from build123d import *

# Parameters (mm, degrees)
BOSS_EXTRUDE1_DEPTH = 3.175
BOSS_EXTRUDE2_DEPTH = 3.175
CUT_EXTRUDE2_DEPTH  = 159.172640977
CIRPATTERN1_COUNT   = 6
SKETCH4_R           = 8.001
CUT_EXTRUDE3_DEPTH  = 3.175
BOSS_EXTRUDE3_DEPTH = 2.54
CIRPATTERN2_COUNT   = 6


with BuildPart() as part:
    # Sketch1 → Boss-Extrude1 (new body)
    with BuildSketch(Plane(origin=(0, 0, 0), x_dir=(1, 0, 0), z_dir=(0, 1, 0))):
        Polygon((55.499999998, -96.128819817), (110.999999996, 0), (55.499999998, 96.128819817), (-55.499999998, 96.128819817), (-110.999999996, 0), (-55.499999998, -96.128819817), align=None)
    extrude(amount=BOSS_EXTRUDE1_DEPTH)

    # Sketch2 → Boss-Extrude2 (add)
    with BuildSketch(Plane(origin=(0, 0, 0), x_dir=(1, 0, 0), z_dir=(0, 1, 0))):
        with BuildLine():
            ThreePointArc((23.622499999, 104.383819817), (24.109685288, 98.980852172), (19.494999999, 96.128819817))
            Line((19.494999999, 96.128819817), (36.004999999, 96.128819817))
            ThreePointArc((36.004999999, 96.128819817), (31.39031471, 98.980852172), (31.877499999, 104.383819817))
            ThreePointArc((31.877499999, 104.383819817), (32.364685288, 109.786787461), (27.749999999, 112.638819817))
            ThreePointArc((27.749999999, 112.638819817), (23.13531471, 109.786787461), (23.622499999, 104.383819817))
        make_face()
    boss_extrude2 = extrude(amount=BOSS_EXTRUDE2_DEPTH)

    # Sketch2<3> → Cut-Extrude2 (cut, through all)
    with BuildSketch(Plane(origin=(0, 0, 0), x_dir=(1, 0, 0), z_dir=(0, 1, 0))):
        with BuildLine():
            Line((-19.494999999, 96.128819817), (-36.004999999, 96.128819817))
            ThreePointArc((-36.004999999, 96.128819817), (-31.39031471, 93.276787461), (-31.877499999, 87.873819817))
            ThreePointArc((-31.877499999, 87.873819817), (-32.364685288, 82.470852172), (-27.749999999, 79.618819817))
            ThreePointArc((-27.749999999, 79.618819817), (-23.13531471, 82.470852172), (-23.622499999, 87.873819817))
            ThreePointArc((-23.622499999, 87.873819817), (-24.109685288, 93.276787461), (-19.494999999, 96.128819817))
        make_face()
    cut_extrude2 = extrude(amount=CUT_EXTRUDE2_DEPTH, mode=Mode.SUBTRACT)

    # CirPattern1: Boss-Extrude2, Cut-Extrude2 ×6 about axis
    cirpattern1_axis = Axis((0, 0, 0), (0, 1, 0))
    add([boss_extrude2.rotate(cirpattern1_axis, i * 360 / CIRPATTERN1_COUNT) for i in range(1, CIRPATTERN1_COUNT)])
    add([cut_extrude2.rotate(cirpattern1_axis, i * 360 / CIRPATTERN1_COUNT) for i in range(1, CIRPATTERN1_COUNT)], mode=Mode.SUBTRACT)

    # Sketch4 → Cut-Extrude3 (cut)
    with BuildSketch(Plane(origin=(0, 3.175, 0), x_dir=(1, 0, 0), z_dir=(0, 1, 0))):
        with Locations(Location((0, 0, 0), (0, 0, 270))):
            Circle(SKETCH4_R)
    extrude(amount=-CUT_EXTRUDE3_DEPTH, mode=Mode.SUBTRACT)

    # Sketch5 → Boss-Extrude3 (add)
    with BuildSketch(Plane(origin=(0, 3.175, 0), x_dir=(1, 0, 0), z_dir=(0, 1, 0))):
        Polygon((-8.429069256, -1.402423789), (-84.749999997, -45.466333697), (-83.249999997, -48.064409908), (-6.929069256, -4.0005), align=None)
        Polygon((-6.929069256, -4.0005), (-83.249999997, -48.064409908), (-81.749999997, -50.66248612), (-5.429069256, -6.598576211), align=None)
    boss_extrude3 = extrude(amount=BOSS_EXTRUDE3_DEPTH)

    # CirPattern2: Boss-Extrude3 ×6 about axis
    cirpattern2_axis = Axis((0, 0, 0), (0, 1, 0))
    for i in range(1, CIRPATTERN2_COUNT):
        add(boss_extrude3.rotate(cirpattern2_axis, i * 360 / CIRPATTERN2_COUNT))


solid = part.part
Verification items for the finished model (mm, model axes). A direction names the side the tool comes from. Coordinates: 2 decimals unless noted, no trailing zeros. Write each loop counter-clockwise with the first axis right and the second up, starting at its lowest first coordinate (ties: lowest second). Pieces come first, ordered by that corner, then holes. Notation, with made-up numbers: (65.5, 21.5) -> (121.5, 21.5) arc R23 cw to (121.5, 30.5) -> close; hole circle Ø4 at (50, 22.25). An arc over 180 degrees is marked (long way). One line per item, written item: value. Start each with the question number.
Q1. Cross-section at A-A on x = 43.5. Enter the section's corners in (y, z) (3 decimals), and give its area (3 significant figures).
Q2. Access from +Z, -Z, +X, -X, +Y, -Y to the whole of each face (thin tool, end or side, straight path). Record for faces 1 (the flat face through (-32, 3.175, 58)), 2 (the flat face through (60.306, 1.565, 87.805)), 3 (the flat face through (-43.055, 4.427, -28.322)).
Q3. Thickness scan on L1, parallel to X at y = 1.7, z = 0; L2, parallel to Z at x = 0, y = 0.7; L3, parallel to Y at x = 90.5, z = -15 (3 decimals). Record the ranges inside material, lowest first. Write a range as from..to.
Q4. Go/stop test with flat-tipped pins: P1, Ø1, axis at x = 46.5, y = 2, coming from the -Z side; P2, Ø3, axis at x = 1, y = 4.5, coming from the +Z side; P3, Ø2, axis at x = -32.5, z = 75.5, coming from the +Y side (3 decimals). Record where each tip stops, or that it passes through.
Q5. Mould release check, pull along Z, two halves, no side actions. Record for faces 4 (the flat face through (-106.194, 1.565, 8.323)), 5 (the flat face through (0, 5.715, 52)), 6 (the flat face through (60.44, 1.57, -87.57)): pulls with the +Z half, pulls with the -Z half, needs draft (parallel to the pull), parting line crosses it, or undercut.
Checked values:
1. outline: (0, -96.129) -> (3.175, -96.129) -> (3.175, -28.579) -> (5.715, -28.579) -> (5.715, -21.651) -> (3.175, -21.651) -> (3.175, 21.651) -> (5.715, 21.651) -> (5.715, 28.579) -> (3.175, 28.579) -> (3.175, 96.129) -> (0, 96.129) -> close
1. area: 646 mm²
2. face 1: +Z, +Y
2. face 2: +Z, +Y, -Y
2. face 3: -Z, +Y
3. L1: x = -111..-8, 8..111
3. L2: z = -96.13..-8, 8..96.13
3. L3: y = 0..3.175
4. P1: stops at z = -96.13
4. P2: stops at z = 96.13
4. P3: stops at y = 3.175
5. face 4: undercut
5. face 5: needs draft
5. face 6: pulls with the -Z half
